from build123d import *

# Parameters (mm, degrees)
SKETCH1_R               = 11.39
BOSS_EXTRUDE1_DEPTH     = 8
SKETCH2_R               = 14
BOSS_EXTRUDE2_DEPTH     = 1.6
SKETCH3_R               = 8.5
BOSS_EXTRUDE3_DEPTH     = 6.3
CUT_EXTRUDE1_DEPTH      = 26.393109302
CUT_EXTRUDE1_DEPTH_BACK = 26.393109302
SKETCH4_R               = 4
SKETCH5_R               = 14
SKETCH5_R_2             = 4
BOSS_EXTRUDE4_DEPTH     = 1.6


with BuildPart() as part:
    # Sketch1 → Boss-Extrude1 (new body)
    with BuildSketch(Plane(origin=(0, 0, 0), x_dir=(1, 0, 0), z_dir=(0, 1, 0))):
        with Locations(Location((0, 0, 0), (0, 0, 270))):
            Circle(SKETCH1_R)
    extrude(amount=BOSS_EXTRUDE1_DEPTH)

    # Sketch2 → Boss-Extrude2 (add)
    with BuildSketch(Plane(origin=(0, 8, 0), x_dir=(1, 0, 0), z_dir=(0, 1, 0))):
        with Locations(Location((0, 0, 0), (0, 0, 270))):
            Circle(SKETCH2_R)
    extrude(amount=BOSS_EXTRUDE2_DEPTH)

    # Sketch3 → Boss-Extrude3 (add)
    with BuildSketch(Plane(origin=(0, 9.6, 0), x_dir=(1, 0, 0), z_dir=(0, 1, 0))):
        with Locations(Location((0, 0, 0), (0, 0, 270))):
            Circle(SKETCH3_R)
    extrude(amount=BOSS_EXTRUDE3_DEPTH)

    # Sketch4 → Cut-Extrude1 (cut, two sides: drawn at the far end of the back side and taken through both)
    with BuildSketch(Plane(origin=(0, 15.9, 0), x_dir=(1, 0, 0), z_dir=(0, 1, 0)).offset(-CUT_EXTRUDE1_DEPTH_BACK)):
        with Locations(Location((0, 0, 0), (0, 0, 270))):
            Circle(SKETCH4_R)
    extrude(amount=CUT_EXTRUDE1_DEPTH + CUT_EXTRUDE1_DEPTH_BACK, mode=Mode.SUBTRACT)

    # Sketch5 → Boss-Extrude4 (add)
    with BuildSketch(Plane.XZ):
        with Locations(Location((0, 0, 0), (0, 0, 90))):
            Circle(SKETCH5_R)
        with Locations(Location((0, 0, 0), (0, 0, 90))):
            Circle(SKETCH5_R_2, mode=Mode.SUBTRACT)
    extrude(amount=BOSS_EXTRUDE4_DEPTH)


solid = part.part
For this review, take the finished solid that the model builds, in its own axes (mm). A direction names the side the tool comes from. Coordinates: 2 decimals unless noted, no trailing zeros. Order: outer loops, then holes, each group sorted by start corner. A loop starts at its lowest first (then second) coordinate and runs counter-clockwise, first axis right, second up. Notation, with made-up numbers: (26.5, 59) -> (61.5, 59) arc R14 ccw to (61.5, 67) -> close; hole circle Ø5 at (-7, 5.25). An arc over 180 degrees is marked (long way). Return JSON: item names as keys, results as strings.
1. For line 1 (Y direction, x = -6.75, z = -11.25); line 2 (X direction, y = 4.5, z = 0); line 3 (X direction, y = 11.75, z = 0), list the stretches that pass through material, from the lowest coordinate up. Write a range as from..to.
Answer block:
{"line 1": "-1.6..0, 8..9.6", "line 2": "-11.39..-4, 4..11.39", "line 3": "-8.5..-4, 4..8.5"}
2. We need section A-A on x = 0. Write out the cut boundary in (y, z), and give its area (3 significant figures).
Answer block:
{"outline": "(-1.6, -14) -> (0, -14) -> (0, -11.39) -> (8, -11.39) -> (8, -14) -> (9.6, -14) -> (9.6, -8.5) -> (15.9, -8.5) -> (15.9, -4) -> (-1.6, -4) -> close; (-1.6, 4) -> (15.9, 4) -> (15.9, 8.5) -> (9.6, 8.5) -> (9.6, 14) -> (8, 14) -> (8, 11.39) -> (0, 11.39) -> (0, 14) -> (-1.6, 14) -> close", "area": "239 mm²"}
3. We need section C-C on y = 5.75. Write out the cut boundary in (x, z), and give its area (3 significant figures).
Answer block:
{"outline": "circle Ø22.78 at (0, 0); hole circle Ø8 at (0, 0)", "area": "357 mm²"}
4. The part is to be moulded in two halves that separate along Z. For faces 1 (the flat face through (-2, 15.9, 4)), 2 (the cylindrical face through (8.428, 12.706, -1.107)), 3 (the cylindrical face through (3.905, 7.273, -0.867)), say which applies: +Z half, -Z half, draft (parallel to the pull), parting line (faces both ways), or undercut.
Answer block:
{"face 1": "draft", "face 2": "parting line", "face 3": "undercut"}
5. We need section B-B on z = 0. Write out the cut boundary in (x, y), and give its area (3 significant figures).
Answer block:
{"outline": "(-14, -1.6) -> (-4, -1.6) -> (-4, 15.9) -> (-8.5, 15.9) -> (-8.5, 9.6) -> (-14, 9.6) -> (-14, 8) -> (-11.39, 8) -> (-11.39, 0) -> (-14, 0) -> close; (4, -1.6) -> (14, -1.6) -> (14, 0) -> (11.39, 0) -> (11.39, 8) -> (14, 8) -> (14, 9.6) -> (8.5, 9.6) -> (8.5, 15.9) -> (4, 15.9) -> close", "area": "239 mm²"}
6. For pin 1 Ø1 at (x, y) = (2.5, 12) entering from -Z; pin 2 Ø2 at (x, y) = (-5, 3) entering from +Z; pin 3 Ø5 at (y, z) = (5, -2.5) entering from +X, all flat-tipped, find the tip position at first contact; note any pin that passes through.
Answer block:
{"pin 1": "z = -8.26", "pin 2": "z = 10.66", "pin 3": "x = 11.39"}
7. We need section D-D on x = -5.5. Write out the cut boundary in (y, z), and give its area (3 significant figures).
Answer block:
{"outline": "(-1.6, -12.87) -> (0, -12.87) -> (0, -9.97) -> (8, -9.97) -> (8, -12.87) -> (9.6, -12.87) -> (9.6, -6.48) -> (15.9, -6.48) -> (15.9, 6.48) -> (9.6, 6.48) -> (9.6, 12.87) -> (8, 12.87) -> (8, 9.97) -> (0, 9.97) -> (0, 12.87) -> (-1.6, 12.87) -> close", "area": "324 mm²"}
8. Machinability: for faces 4 (the flat face through (11.34, 0, -2.14)), 5 (the cylindrical face through (13.67, -0.79, -3.03)), 6 (the flat face through (-9, 9.6, 0)), which of the approach directions +Z, -Z, +X, -X, +Y, -Y give a long, thin tool a straight path to every point of the face, cutting with its end or side? Answer none if there is none.
Answer block:
{"face 4": "none", "face 5": "+Y, -Y", "face 6": "+Y"}
